Design review of the part built by this model. Coordinates are the model's own, in mm. A direction names the side the tool comes from. Round coordinates to 2 decimals unless told otherwise and drop trailing zeros. Order: outer loops, then holes, each group sorted by start corner. A loop starts at its lowest first (then second) coordinate and runs counter-clockwise, first axis right, second up. Notation, with made-up numbers: (36, 86) - (93, 86) arc R16 cw to (93, 94) - close; hole circle Ø7 at (53.25, -23). An arc over 180 degrees is marked (long way). Write item = value, one per line.
from build123d import *

# Parameters (mm, degrees)
F0_R     = 10
F0_R_2   = 8
F0_R_3   = 2
F1_DEPTH = 1
F2_DEPTH = 4
F3_DEPTH = 2


with BuildPart() as f1:
    # F0 (on Top) → F1 (new body)
    with BuildSketch(Plane.XY):
        Circle(F0_R)
        Circle(F0_R_2, mode=Mode.SUBTRACT)
        Circle(F0_R_2)
        with BuildLine():
            ThreePointArc((6.3245553203, 3), (6.8290514437, 1.5375488216), (7, 0))
            ThreePointArc((7, 0), (6.8290514437, -1.5375488216), (6.3245553203, -3))
            ThreePointArc((6.3245553203, -3), (4.7537534147, -5.1382709614), (2.5, -6.5383484153))
            ThreePointArc((2.5, -6.5383484153), (-2.6051455289, -6.4971699049), (-6.3245553203, -3))
            ThreePointArc((-6.3245553203, -3), (-7, 0), (-6.3245553203, 3))
            ThreePointArc((-6.3245553203, 3), (-2.6051455289, 6.4971699049), (2.5, 6.5383484153))
            ThreePointArc((2.5, 6.5383484153), (4.7537534147, 5.1382709614), (6.3245553203, 3))
        make_face(mode=Mode.SUBTRACT)
        with BuildLine():
            Line((2.5, -3), (2.5, 3))
            Line((2.5, 3), (-6.3245553203, 3))
            ThreePointArc((-6.3245553203, 3), (-7, 0), (-6.3245553203, -3))
            Line((-6.3245553203, -3), (2.5, -3))
        make_face()
        Circle(F0_R_3, mode=Mode.SUBTRACT)
        with BuildLine():
            Line((2.5, 3), (2.5, 6.5383484153))
            ThreePointArc((2.5, 6.5383484153), (-2.6051455289, 6.4971699049), (-6.3245553203, 3))
            Line((-6.3245553203, 3), (2.5, 3))
        make_face()
        with BuildLine():
            ThreePointArc((-6.3245553203, -3), (-2.6051455289, -6.4971699049), (2.5, -6.5383484153))
            Line((2.5, -6.5383484153), (2.5, -3))
            Line((2.5, -3), (-6.3245553203, -3))
        make_face()
        with BuildLine():
            ThreePointArc((6.3245553203, -3), (6.8290514437, -1.5375488216), (7, 0))
            ThreePointArc((7, 0), (6.8290514437, 1.5375488216), (6.3245553203, 3))
            Line((6.3245553203, 3), (2.5, 3))
            Line((2.5, 3), (2.5, -3))
            Line((2.5, -3), (6.3245553203, -3))
        make_face()
        with BuildLine():
            Line((2.5, 3), (6.3245553203, 3))
            ThreePointArc((6.3245553203, 3), (4.7537534147, 5.1382709614), (2.5, 6.5383484153))
            Line((2.5, 6.5383484153), (2.5, 3))
        make_face()
        with BuildLine():
            ThreePointArc((2.5, -6.5383484153), (4.7537534147, -5.1382709614), (6.3245553203, -3))
            Line((6.3245553203, -3), (2.5, -3))
            Line((2.5, -3), (2.5, -6.5383484153))
        make_face()
    extrude(amount=F1_DEPTH)

    # F0 (on Top) → F2 (join)
    with BuildSketch(Plane.XY):
        Circle(F0_R_2)
        with BuildLine():
            ThreePointArc((6.3245553203, 3), (6.8290514437, 1.5375488216), (7, 0))
            ThreePointArc((7, 0), (6.8290514437, -1.5375488216), (6.3245553203, -3))
            ThreePointArc((6.3245553203, -3), (4.7537534147, -5.1382709614), (2.5, -6.5383484153))
            ThreePointArc((2.5, -6.5383484153), (-2.6051455289, -6.4971699049), (-6.3245553203, -3))
            ThreePointArc((-6.3245553203, -3), (-7, 0), (-6.3245553203, 3))
            ThreePointArc((-6.3245553203, 3), (-2.6051455289, 6.4971699049), (2.5, 6.5383484153))
            ThreePointArc((2.5, 6.5383484153), (4.7537534147, 5.1382709614), (6.3245553203, 3))
        make_face(mode=Mode.SUBTRACT)
    extrude(amount=F2_DEPTH)

    # F0 (on Top) → F3 (join)
    with BuildSketch(Plane.XY):
        with BuildLine():
            Line((2.5, 3), (2.5, 6.5383484153))
            ThreePointArc((2.5, 6.5383484153), (-2.6051455289, 6.4971699049), (-6.3245553203, 3))
            Line((-6.3245553203, 3), (2.5, 3))
        make_face()
        with BuildLine():
            Line((2.5, 3), (6.3245553203, 3))
            ThreePointArc((6.3245553203, 3), (4.7537534147, 5.1382709614), (2.5, 6.5383484153))
            Line((2.5, 6.5383484153), (2.5, 3))
        make_face()
        with BuildLine():
            ThreePointArc((6.3245553203, -3), (6.8290514437, -1.5375488216), (7, 0))
            ThreePointArc((7, 0), (6.8290514437, 1.5375488216), (6.3245553203, 3))
            Line((6.3245553203, 3), (2.5, 3))
            Line((2.5, 3), (2.5, -3))
            Line((2.5, -3), (6.3245553203, -3))
        make_face()
        with BuildLine():
            ThreePointArc((2.5, -6.5383484153), (4.7537534147, -5.1382709614), (6.3245553203, -3))
            Line((6.3245553203, -3), (2.5, -3))
            Line((2.5, -3), (2.5, -6.5383484153))
        make_face()
        with BuildLine():
            ThreePointArc((-6.3245553203, -3), (-2.6051455289, -6.4971699049), (2.5, -6.5383484153))
            Line((2.5, -6.5383484153), (2.5, -3))
            Line((2.5, -3), (-6.3245553203, -3))
        make_face()
    extrude(amount=F3_DEPTH)


solid = f1.part
Item 1: Take a section at C-C, the plane y = -6.25. State the section outline as (x, z) points, and give its area (3 significant figures).
Data:
outline = (-7.81, 0) - (7.81, 0) - (7.81, 1) - (4.99, 1) - (4.99, 4) - (3.15, 4) - (3.15, 2) - (-3.15, 2) - (-3.15, 4) - (-4.99, 4) - (-4.99, 1) - (-7.81, 1) - close
area = 33.0 mm2
Item 2: For faces 4 (the face through (4, -6, 4)), 5 (the face through (-1.73, -7.81, 2.48)), list the 3-axis set-ups (+Z, -Z, +X, -X, +Y, -Y) from which the entire face can be reached by the end or side of a thin tool; tool diameter is ignored.
Data:
face_4 = +Z, +X, -X, +Y, -Y
face_5 = +Z
Item 3: Insertion check: P1, Ø5, axis at x = 0, y = 0, coming from the -Z side; P2, Ø6.5, axis at x = -3, y = 0.5, coming from the +Z side; P3, Ø2, axis at x = 1, z = 3.5, coming from the -Y side; P4, Ø0.5, axis at y = 0, z = 1.5, coming from the -X side. Each pin has a flat end and moves straight along its axis. Give the tip position at first contact, or say it passes through.
Data:
P1 = 0
P2 = 2
P3 = -8
P4 = -8
Item 4: Take a section at D-D, the plane x = 2.25. State the section outline as (y, z) points, and give its area (3 significant figures).
Data:
outline = (-9.74, 0) - (9.74, 0) - (9.74, 1) - (7.68, 1) - (7.68, 4) - (6.63, 4) - (6.63, 2) - (3, 2) - (3, 1) - (-3, 1) - (-3, 2) - (-6.63, 2) - (-6.63, 4) - (-7.68, 4) - (-7.68, 1) - (-9.74, 1) - close
area = 33.0 mm2
Item 5: Take a section at B-B, the plane z = 2.4. State the section outline as (x, y) points, and give its area (3 significant figures).
Data:
outline = circle Ø16 at (0, 0); hole circle Ø14 at (0, 0)
area = 47.1 mm2
Item 6: Take a section at A-A, the plane x = 0. State the section outline as (y, z) points, and give its area (3 significant figures).
Data:
outline = (-10, 0) - (-2, 0) - (-2, 1) - (-3, 1) - (-3, 2) - (-7, 2) - (-7, 4) - (-8, 4) - (-8, 1) - (-10, 1) - close; (2, 0) - (10, 0) - (10, 1) - (8, 1) - (8, 4) - (7, 4) - (7, 2) - (3, 2) - (3, 1) - (2, 1) - close
area = 30.0 mm2
Item 7: For line 1 along Y through (x, z) = (0, 0.55); line 2 along Z through (x, y) = (9.25, 0.5); line 3 along Y through (x, z) = (0, 2.1), list the stretches that pass through material, from the lowest coordinate up. Write a range as [from, to].
Data:
line_1 = [-10, -2], [2, 10]
line_2 = [0, 1]
line_3 = [-8, -7], [7, 8]
Item 8: The part is to be moulded in two halves that separate along X. For faces 1 (the face through (-2.17, -9.76, 0.49)), 2 (the face through (-1.9, -3, 1.5)), 3 (the face through (-0.1, 2.4, 0)), say which applies: +X half, -X half, draft (parallel to the pull), parting line (faces both ways), or undercut.
Data:
face_1 = parting line
face_2 = undercut
face_3 = draft
